```python
from build123d import *

# Parameters (mm, degrees)
F0_R     = 2
F1_DEPTH = 14.8
F2_DEPTH = 2.8
F5_SIZE  = 0.3


with BuildPart() as f1:
    # F0 (on Top) → F1 (new body)
    with BuildSketch(Plane.XY):
        Circle(F0_R)
    extrude(amount=F1_DEPTH)

    # F0 (on Top) → F2 (join)
    with BuildSketch(Plane.XY):
        Polygon((3.5, 2.020726), (0, 4.041452), (-3.5, 2.020726), (-3.5, -2.020726), (0, -4.041452), (3.5, -2.020726), align=None)
        Circle(F0_R, mode=Mode.SUBTRACT)
    extrude(amount=F2_DEPTH)

    # F3 (on Right) → F4 (revolve, cut)
    with BuildSketch(Plane.YZ):
        with BuildLine():
            add(Edge.make_bspline(
                [(2.858781, 0), (3.303965, 0), (3.651425, 0), (4.042318, 0.235874)],
                knots=[0, 0, 0, 0, 1.206813, 1.206813, 1.206813, 1.206813], degree=3))
            Line((2.858781, 0), (4.043203, 0))
            Line((4.043203, 0), (4.042318, 0.235874))
        make_face()
    revolve(axis=Axis((0, 0, 0), (0, 0, -1)), mode=Mode.SUBTRACT)

    # F5
    f5_edges = [f1.edges().sort_by_distance(p)[0] for p in [
        (-2, 0, 14.8),
    ]]
    chamfer(f5_edges, length=F5_SIZE)


solid = f1.part
```
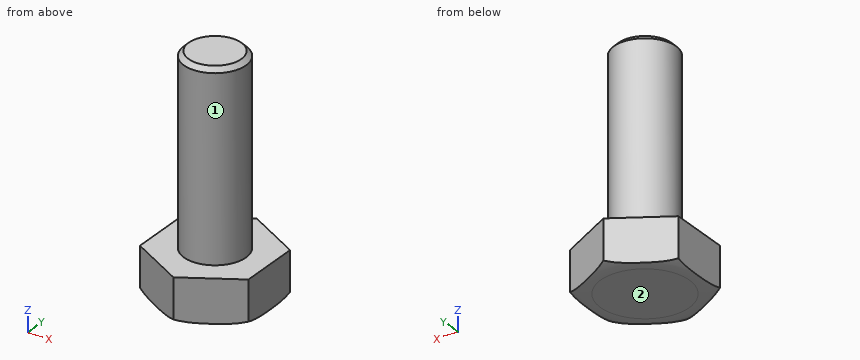
Read the model definition and answer for the solid it produces. Units are mm, in the model's axes. Face numbers are marked on the shaded views. A direction names the side the tool comes from. Give positions to 0.01 mm unless a question says otherwise; leave off trailing zeros. Write each loop counter-clockwise with the first axis right and the second up, starting at its lowest first coordinate (ties: lowest second). Pieces come first, ordered by that corner, then holes. Notation, with made-up numbers: (86.25, 9.25) - (136.25, 9.25) arc R26 cw to (136.25, 28.25) - close; hole circle Ø6 at (60, 81.25). An arc over 180 degrees is marked (long way). Write item = value, one per line. Start each with the question number.
Item 1: Find section A-A (z = 1). Give the vertices of the cut face in (x, y), then the cut area to 3 significant figures.
Item 2: A tool of negligible diameter and unlimited length cuts with its end or side. For the marked faces 1 and 2, from which of +Z, -Z, +X, -X, +Y, -Y can it reach the whole face along a straight path? Write none if from no direction.
Item 3: Each of these flat-tipped pins is pushed along its axis until it touches: P1, Ø2, axis at x = 0, z = 3, coming from the +Y side; P2, Ø3, axis at y = 0.5, z = 1.5, coming from the -X side; P3, Ø0.8, axis at y = 0.5, z = 2, coming from the +X side; P4, Ø1.5, axis at y = 3, z = 10, coming from the -X side. Where does it stop, or does it pass through?
Item 4: Find the intervals of material crossed by probe 1 along Z at (x, y) = (0.5, -2.5); probe 2 along X at (y, z) = (1, 2.5); probe 3 along Y at (x, z) = (-0.75, 10), in increasing order. Write a range as [from, to].
Item 5: Find section B-B (z = 7). Give the vertices of the cut face in (x, y).
Response:
q1.outline = (-3.5, -2.02) - (0, -4.04) - (3.5, -2.02) - (3.5, 2.02) - (0, 4.04) - (-3.5, 2.02) - close
q1.area = 42.4 mm²
q2.face_1 = +Z
q2.face_2 = -Z, +X, -X, +Y, -Y
q3.P1 = 4.04
q3.P2 = -3.5
q3.P3 = 3.5
q3.P4 = through
q4.probe_1 = [0, 2.8]
q4.probe_2 = [-3.5, 3.5]
q4.probe_3 = [-1.85, 1.85]
q5.outline = circle Ø4 at (0, 0)
